The model under review builds one solid part; all positions refer to its coordinate system, in mm. A direction names the side the tool comes from. Coordinates: 2 decimals unless noted, no trailing zeros. Order: outer loops, then holes, each group sorted by start corner. A loop starts at its lowest first (then second) coordinate and runs counter-clockwise, first axis right, second up. Notation, with made-up numbers: M -27,-2.75 L 32,-2.75 A13 cw 32,16.25 Z; hole C 76,-27 d3. An arc over 180 degrees is marked long. Answer as CSV lines item,"result". Start each with the question number.
Q1. Machinability: for faces 1 (the face through (21.04, -21.57, 12.46)), 2 (the face through (13.91, -10.02, 17.18)), 3 (the face through (14.646, -21.572, 16.703)), which of the approach directions +Z, -Z, +X, -X, +Y, -Y give a long, thin tool a straight path to every point of the face, cutting with its end or side? Answer none if there is none.
Q2. Consider section C-C on z = 11. Write out the cut boundary in (x, y).
Q3. The part is to be moulded in two halves that separate along X. For faces 4 (the face through (31.76, -11.27, 8.43)), 5 (the face through (-9, -22.8, 22.6)), 6 (the face through (20, -22.86, 15)), say which applies: +X half, -X half, draft (parallel to the pull), parting line (faces both ways), or undercut.
Q4. Consider section D-D on x = -22. Write out the cut boundary in (y, z), and give its area (3 significant figures).
Q5. For P1, Ø12, axis at y = -12.5, z = 26.5, coming from the -X side; P2, Ø1.5, axis at y = -17, z = 19.5, coming from the -X side; P3, Ø1, axis at y = -18, z = 6, coming from the -X side, all flat-tipped, find the tip position at first contact; note any pin that passes through.
Q6. Wall thickness on L1, parallel to X at y = -21.5, z = 24; L2, parallel to Y at x = 3, z = 0; L3, parallel to Y at x = 19, z = 16.5: over which ranges is each line inside the solid? List them lowest first. Write a range as [from, to].
Q7. Consider section A-A on z = 22.5. Write out the cut boundary in (x, y).
Q8. Consider section B-B on y = -13.25. Write out the cut boundary in (x, z).
from build123d import *

# Parameters (mm, degrees)
F1_DEPTH = 25.4
F2_DEPTH = 5.08
F4_DEPTH = 5.08
F6_DEPTH = 5.08
F7_DEPTH = 2.54


with BuildPart() as f1:
    # F0 (on Front) → F1 (new body)
    with BuildSketch(Plane.XZ):
        Polygon((8.4221055731, 9.6252635121), (-8.1213163212, 34.5907881856), (-38.5010540485, -7.2189471684), (43.9152643085, -7.2189471684), (19.2508431466, 24.5281786139), align=None)
    extrude(amount=F1_DEPTH)

    # F2 (cut): a face of the model
    f2_faces = [f1.faces().sort_by_distance(p)[0] for p in [
        (1.3839184885, -25.4, 6.2098147026),
    ]]
    extrude(f2_faces, amount=-F2_DEPTH, mode=Mode.SUBTRACT)

    # F3 (on face) → F4 (join)
    with BuildSketch(Plane.XZ.offset(20.32)):
        Polygon((0, 15.509402017), (-8.1213163212, 34.5907881856), (-15.716250753, 24.1383543471), (-23.3111851849, 13.6859205086), (-12.633157894, 24.1383543471), (-9.9049633738, 21.351277577), (-8.1213163212, 23.8059995994), align=None)
    extrude(amount=F4_DEPTH)

    # F5 (on face) → F6 (join)
    with BuildSketch(Plane.XZ.offset(20.32)):
        Polygon((31.5830537275, 8.6546157228), (19.2508431466, 24.5281786139), (9.9095513281, 8.6546157228), (16.3856597612, 13.6859205086), (19.2508431466, 9.9979629957), (22.8732819398, 14.98329923), align=None)
    extrude(amount=F6_DEPTH)

    # F7 (cut): a face of the model
    f7_faces = [f1.faces().sort_by_distance(p)[0] for p in [
        (19.8070463601, -25.4, 16.0557240809),
    ]]
    extrude(f7_faces, amount=-F7_DEPTH, mode=Mode.SUBTRACT)


solid = f1.part
Evaluation:
1,face 1,"-Z, -Y"
1,face 2,"+Z, +Y, -Y"
1,face 3,"+Z, -Y"
2,outline,"M -25.26,-20.32 L 7.51,-20.32 L 7.51,0 L -25.26,0 Z; M 9.42,-20.32 L 11.29,-20.32 L 11.29,-22.86 L 12.93,-22.86 L 12.93,-20.32 L 18.47,-20.32 L 18.47,-22.86 L 19.98,-22.86 L 19.98,-20.32 L 28.36,-20.32 L 28.36,-22.86 L 29.76,-22.86 L 29.76,0 L 9.42,0 Z"
3,face 4,"+X half"
3,face 5,"undercut"
3,face 6,"draft"
4,outline,"M -25.4,14.97 L -20.32,14.97 L -20.32,-7.22 L 0,-7.22 L 0,15.49 L -25.4,15.49 Z"
4,area,"464 mm²"
5,P1,"stops at x = -18.36"
5,P2,"stops at x = -19.63"
5,P3,"stops at x = -29.26"
6,L1,"x = [-15.82, -12.77], [-12.5, -3.61], [18.94, 19.66]"
6,L2,"y = [-20.32, 0]"
6,L3,"y = [-22.86, 0]"
7,outline,"M -16.91,-25.4 L -14.31,-25.4 L -14.31,-20.32 L -11.03,-20.32 L -11.03,-25.4 L -9.07,-25.4 L -9.07,-20.32 L -6.84,-20.32 L -6.84,-25.4 L -2.98,-25.4 L -2.98,-20.32 L -0.11,-20.32 L -0.11,0 L -16.91,0 Z; M 17.78,-20.32 L 18.06,-20.32 L 18.06,-22.86 L 20.83,-22.86 L 20.83,0 L 17.78,0 Z"
8,outline,"M -38.5,-7.22 L 43.92,-7.22 L 19.25,24.53 L 8.42,9.63 L -8.12,34.59 Z"
